Read the model definition and answer for the solid it produces. Units are mm, in the model's axes. Face numbers are marked on the shaded views. A direction names the side the tool comes from. Round coordinates to 2 decimals unless told otherwise and drop trailing zeros. Order: outer loops, then holes, each group sorted by start corner. A loop starts at its lowest first (then second) coordinate and runs counter-clockwise, first axis right, second up. Notation, with made-up numbers: (-23.5, -29.5) - (7.5, -29.5) arc R20 ccw to (7.5, -15.5) - close; hole circle Ø5 at (65, 89.25). An arc over 180 degrees is marked (long way). Answer as a JSON object with one key per item and string values. Group by question number.
Q1. The mould has two halves that part along Z. Classify the marked faces 1, 2 and 3: pulls with the +Z half, pulls with the -Z half, needs draft (parallel to the pull), parting line crosses it, or undercut.
Q2. A tool of negligible diameter and unlimited length cuts with its end or side. For the marked faces 4, 5, 6 and 7, from which of +Z, -Z, +X, -X, +Y, -Y can it reach the whole face along a straight path? Write none if from no direction.
Q3. Consider line 1 (Z direction, x = 53.9, y = 6.5); line 2 (Z direction, x = -8, y = 6); line 3 (X direction, y = 26, z = 4.5). Determine where each line is inside the solid, lowest interval first.
Q4. Given pin 1 Ø5 at (x, z) = (54, -1) entering from +Y; pin 2 Ø1.5 at (y, z) = (30.5, 29) entering from +X; pin 3 Ø20.5 at (x, z) = (17.5, 18.5) entering from -Y, each flat-ended and moving along its own axis, determine where each tip first touches the part or whether it passes through.
Q5. A cutting plane is placed at D-D on z = 23.5. Determine the outline of the cut face in (x, y).
Q6. A cutting plane is placed at C-C on x = 53.9. Determine the outline of the cut face in (y, z).
Q7. A cutting plane is placed at B-B on z = 14. Determine the outline of the cut face in (x, y), and give its area (3 significant figures).
```python
from build123d import *
from OCP.BRepFilletAPI import BRepFilletAPI_MakeFillet

# Parameters (mm, degrees)
SKETCH_1_W           = 71.9
SKETCH_1_H           = 40.1
SKETCH_1_W_2         = 4
SKETCH_1_H_2         = 1.4
SKETCH_1_H_3         = 0.9
EXTRUDE_1_DEPTH      = 35
SKETCH_4_W           = 8.4
SKETCH_4_H           = 4.4
SKETCH_4_W_2         = 30
SKETCH_4_H_2         = 2
CUT_EXTRUDE_2_DEPTH  = 77.710233998
SKETCH_5_W           = 71.9
SKETCH_5_H           = 40.1
EXTRUDE_2_DEPTH      = 3
SKETCH_6_W           = 47
SKETCH_6_H           = 0.9
CUT_EXTRUDE_3_DEPTH  = 79.124643999
SKETCH_7_R           = 1.6
CUT_EXTRUDE_4_DEPTH  = 79.124643999
SKETCH_10_W          = 10
SKETCH_10_H          = 39.2
SKETCH_10_H_2        = 40.1
CUT_EXTRUDE_6_DEPTH  = 35
CHAMFER_1_SIZE       = 10
CHAMFER_1_SIZE_2     = 11.917535926
SKETCH_8_R           = 3
CUT_EXTRUDE_5_DEPTH  = 35
SKETCH_11_W          = 17
SKETCH_11_H          = 32
CUT_EXTRUDE_7_DEPTH  = 2
CUT_EXTRUDE_8_DEPTH  = 79.124643999
FILLET_2_R1          = 2
FILLET_2_R2          = 3
SKETCH_13_W          = 24.9
SKETCH_13_H          = 1
EXTRUDE_3_DEPTH      = 38
SKETCH_14_W          = 11.9
SKETCH_14_H          = 1
CUT_EXTRUDE_9_DEPTH  = 35
CUT_EXTRUDE_10_REACH = 80.571
SKETCH_15_W          = 10
SKETCH_15_H          = 1
FILLET_3_R           = 3
FILLET_4_R           = 3
SKETCH_16_W          = 14.9
SKETCH_16_H          = 5.6
CUT_EXTRUDE_11_DEPTH = 35
FILLET_5_R           = 3


# Some blends are built 0.0001 mm under size
with BuildPart() as part:
    # 草图1 → 凸台-拉伸1 (new body)
    # profile 1 of 3: a face of its own
    with BuildSketch(Plane(origin=(0, 0, 0), x_dir=(1, 0, 0), z_dir=(0, 1, 0))):
        with Locations((22.95, -14.45)):
            Rectangle(SKETCH_1_W, SKETCH_1_H)
        Polygon((45.9, -32.5), (0, -32.5), (0, 0), (26.7, 0), (26.7, 2.6), (41.1, 2.6), (41.1, 0), (45.9, 0), align=None, mode=Mode.SUBTRACT)
    # profile 2 of 3: a face of its own
    with BuildSketch(Plane(origin=(0, 0, 0), x_dir=(1, 0, 0), z_dir=(0, 1, 0))):
        with Locations((2, -0.7)):
            Rectangle(SKETCH_1_W_2, SKETCH_1_H_2)
    # profile 3 of 3: a face of its own
    with BuildSketch(Plane(origin=(0, 0, 0), x_dir=(1, 0, 0), z_dir=(0, 1, 0))):
        with Locations((2, -32.05)):
            Rectangle(SKETCH_1_W_2, SKETCH_1_H_3)
    extrude(amount=EXTRUDE_1_DEPTH)

    # 草图4 → 切除-拉伸2 (cut, through all)
    with BuildSketch(Plane(origin=(0, 35, 0), x_dir=(1, 0, 0), z_dir=(0, 1, 0))):
        with Locations((10.12, 0.8)):
            Rectangle(SKETCH_4_W, SKETCH_4_H)
        with Locations((19, -33.5)):
            Rectangle(SKETCH_4_W_2, SKETCH_4_H_2)
    extrude(amount=-CUT_EXTRUDE_2_DEPTH, mode=Mode.SUBTRACT)

    # 草图5 → 凸台-拉伸2 (add)
    with BuildSketch(Plane(origin=(0, 35, 0), x_dir=(1, 0, 0), z_dir=(0, 1, 0))):
        with Locations((22.95, -14.45)):
            Rectangle(SKETCH_5_W, SKETCH_5_H)
    extrude(amount=EXTRUDE_2_DEPTH)

    # 草图6 → 切除-拉伸3 (cut, through all)
    with BuildSketch(Plane.XZ):
        with Locations((10.5, 34.05)):
            Rectangle(SKETCH_6_W, SKETCH_6_H)
    extrude(amount=-CUT_EXTRUDE_3_DEPTH, mode=Mode.SUBTRACT)

    # 草图7 → 切除-拉伸4 (cut, through all)
    with BuildSketch(Plane.XZ):
        with Locations(Location((-8, 27.5, 0), (0, 0, 270))):
            Circle(SKETCH_7_R)
        with Locations(Location((53.9, 27.5, 0), (0, 0, 270))):
            Circle(SKETCH_7_R)
        with Locations(Location((-8, -0.6, 0), (0, 0, 270))):
            Circle(SKETCH_7_R)
        with Locations(Location((53.9, -0.6, 0), (0, 0, 270))):
            Circle(SKETCH_7_R)
    extrude(amount=-CUT_EXTRUDE_4_DEPTH, mode=Mode.SUBTRACT)

    # 草图10 → 切除-拉伸6 (cut)
    with BuildSketch(Plane(origin=(0, 38, 0), x_dir=(1, 0, 0), z_dir=(0, 1, 0))):
        with Locations((-8, -14)):
            Rectangle(SKETCH_10_W, SKETCH_10_H)
        with Locations((53.9, -14.45)):
            Rectangle(SKETCH_10_W, SKETCH_10_H_2)
    extrude(amount=-CUT_EXTRUDE_6_DEPTH, mode=Mode.SUBTRACT)

    # 倒角1
    # the kernel refuses this chamfer: 11.917535926, 10 mm, written as the material it adds along each edge
    with BuildSketch(Plane(origin=(48.9, 3, -5.6), x_dir=(0.9993728857116146, -0.03540953691366307, 0), z_dir=(0, 0, 1))) as chamfer_1_piece_1_section:
        Polygon((CHAMFER_1_SIZE * 0.999372885712, CHAMFER_1_SIZE * 0.0354095369137), (-CHAMFER_1_SIZE_2 * 0.0354095369135, CHAMFER_1_SIZE_2 * 0.999372885707), (0, 0), align=None)
    chamfer_1_piece_1 = extrude(amount=40.1, mode=Mode.PRIVATE)
    chamfer_1_piece_1 = split(chamfer_1_piece_1, bisect_by=Plane(origin=(58.9, 6.996958781, 14.489120948), z_dir=(-1, 0, 0)), keep=Keep.TOP, mode=Mode.PRIVATE)
    chamfer_1_piece_1 = chamfer_1_piece_1 - Plane(origin=(53.9, 6.996958781, 27.5), x_dir=(0, 0, -1), z_dir=(0, -1, 0)) * Cylinder(1.6, 128, mode=Mode.PRIVATE)
    chamfer_1_piece_1 = chamfer_1_piece_1 - Plane(origin=(53.9, 6.996958781, -0.6), x_dir=(0, 0, -1), z_dir=(0, -1, 0)) * Cylinder(1.6, 128, mode=Mode.PRIVATE)
    add(chamfer_1_piece_1)
    with BuildSketch(Plane(origin=(-3, 3, -5.6), x_dir=(-0.9993728857116146, -0.03540953691366305, 0), z_dir=(0, 0, 1))) as chamfer_1_piece_2_section:
        Polygon((CHAMFER_1_SIZE * 0.999372885712, -CHAMFER_1_SIZE * 0.0354095369137), (-CHAMFER_1_SIZE_2 * 0.0354095369135, -CHAMFER_1_SIZE_2 * 0.999372885707), (0, 0), align=None)
    chamfer_1_piece_2 = extrude(amount=39.2, mode=Mode.PRIVATE)
    chamfer_1_piece_2 = split(chamfer_1_piece_2, bisect_by=Plane(origin=(-13, 6.997914765, 14.022030522), z_dir=(1, 0, 0)), keep=Keep.TOP, mode=Mode.PRIVATE)
    chamfer_1_piece_2 = chamfer_1_piece_2 - Plane(origin=(-8, 6.997914765, 27.5), x_dir=(0, 0, -1), z_dir=(0, -1, 0)) * Cylinder(1.6, 127, mode=Mode.PRIVATE)
    chamfer_1_piece_2 = chamfer_1_piece_2 - Plane(origin=(-8, 6.997914765, -0.6), x_dir=(0, 0, -1), z_dir=(0, -1, 0)) * Cylinder(1.6, 127, mode=Mode.PRIVATE)
    add(chamfer_1_piece_2)

    # 草图8 → 切除-拉伸5 (cut)
    with BuildSketch(Plane(origin=(0, 38, 0), x_dir=(1, 0, 0), z_dir=(0, 1, 0))):
        with Locations(Location((-8, 0.6, 0), (0, 0, 270))):
            Circle(SKETCH_8_R)
        with Locations(Location((53.9, 0.6, 0), (0, 0, 270))):
            Circle(SKETCH_8_R)
        with Locations(Location((53.9, -27.5, 0), (0, 0, 270))):
            Circle(SKETCH_8_R)
        with Locations(Location((-8, -27.5, 0), (0, 0, 270))):
            Circle(SKETCH_8_R)
    extrude(amount=-CUT_EXTRUDE_5_DEPTH, mode=Mode.SUBTRACT)

    # 草图11 → 切除-拉伸7 (cut)
    with BuildSketch(Plane.XY.offset(33.6)):
        with Locations((-4.5, 16)):
            Rectangle(SKETCH_11_W, SKETCH_11_H)
    extrude(amount=-CUT_EXTRUDE_7_DEPTH, mode=Mode.SUBTRACT)

    # 草图12 → 切除-拉伸8 (cut, through all)
    with BuildSketch(Plane(origin=(0, 38, 0), x_dir=(1, 0, 0), z_dir=(0, 1, 0))):
        Polygon((3, -2.4), (3, -25.6), (32.9, -2.4), align=None)
        Polygon((42.9, -2.4), (13, -25.6), (42.9, -25.6), align=None)
    extrude(amount=-CUT_EXTRUDE_8_DEPTH, mode=Mode.SUBTRACT)

    # 圆角2: one fillet with a radius per group of edges: ONE call of the kernel's fillet builder (fillet() takes one radius for all edges)
    fillet_2_edges_1 = [part.edges().sort_by_distance(p)[0] for p in [
        (13, 36.5, 25.6),
        (32.9, 36.5, 2.4),
    ]]
    fillet_2_edges_2 = [part.edges().sort_by_distance(p)[0] for p in [
        (3, 36.5, 25.6),
        (42.9, 36.5, 25.6),
        (42.9, 36.5, 2.4),
        (3, 36.5, 2.4),
    ]]
    fillet_2 = BRepFilletAPI_MakeFillet(part.part.solid().wrapped)
    for e in fillet_2_edges_1:
        fillet_2.Add(FILLET_2_R1, e.wrapped)
    for e in fillet_2_edges_2:
        fillet_2.Add(FILLET_2_R2, e.wrapped)
    add(Compound.cast(fillet_2.Shape()), mode=Mode.REPLACE)

    # 草图13 → 凸台-拉伸3 (add)
    with BuildSketch(Plane.XZ):
        with Locations((46.45, 35)):
            Rectangle(SKETCH_13_W, SKETCH_13_H)
    extrude(amount=-EXTRUDE_3_DEPTH)

    # 草图14 → 切除-拉伸9 (cut)
    with BuildSketch(Plane.XZ):
        with Locations((39.95, 33)):
            Rectangle(SKETCH_14_W, SKETCH_14_H)
    extrude(amount=-CUT_EXTRUDE_9_DEPTH, mode=Mode.SUBTRACT)

    # 切除-拉伸10: up to this face of the body (flat: up to its plane)
    cut_extrude_10_end = Plane(part.part.faces().sort_by_distance((53.9, 8.958767963, 14.614170269))[0])
    # 草图15 → 切除-拉伸10 (cut, up to the picked face)
    with BuildSketch(Plane(origin=(0, 38, 0), x_dir=(1, 0, 0), z_dir=(0, 1, 0)), mode=Mode.PRIVATE) as cut_extrude_10_sk1:
        with Locations((53.9, -35)):
            Rectangle(SKETCH_15_W, SKETCH_15_H)
    cut_extrude_10_tool1 = split(extrude(cut_extrude_10_sk1.sketch, amount=-CUT_EXTRUDE_10_REACH, mode=Mode.PRIVATE), bisect_by=cut_extrude_10_end, keep=Keep.BOTH, mode=Mode.PRIVATE)
    add(cut_extrude_10_tool1.solids().sort_by(Axis((53.9, 38, 35), (0, -1, 0)))[0], mode=Mode.SUBTRACT)

    # 圆角3
    fillet_3_edges = [part.edges().sort_by_distance(p)[0] for p in [
        (-3, 26.458767963, -5.6),
        (48.9, 26.458767963, -5.6),
        (48.9, 26.458767963, 35.5),
        (-3, 23.458767963, 31.6),
    ]]
    fillet(fillet_3_edges, radius=FILLET_3_R - 0.0001)  # a hair under: the kernel refuses the full size

    # 圆角4
    # the kernel refuses this fillet: 3 mm, written as the material it adds along each edge
    with BuildSketch(Plane(origin=(34, 35, 33.6), x_dir=(0, 0, 1), z_dir=(0, 1, 0))) as fillet_4_piece_1:
        with BuildLine():
            CenterArc((3, -2.791057147), FILLET_4_R, 111.510188267, 68.489811733)
            Line((0, -2.791057147), (-0.06, -2.791057147))
            Line((-0.06, -2.791057147), (-0.06, 0))
            Line((-0.06, 0), (0, 0.06))
            ThreePointArc((0, 0.06), (0.95, 0.06), (1.878, 0.055821143))
            Line((1.878, 0.055821143), (1.9, 0))
        make_face()
    extrude(amount=3)

    # 草图16 → 切除-拉伸11 (cut)
    with BuildSketch(Plane.XZ):
        with Locations((24.45, -2.8)):
            Rectangle(SKETCH_16_W, SKETCH_16_H)
    extrude(amount=-CUT_EXTRUDE_11_DEPTH, mode=Mode.SUBTRACT)

    # 圆角5
    fillet_5_edges = [part.edges().sort_by_distance(p)[0] for p in [
        (31.9, 17.5, -5.6),
        (17, 17.5, -5.6),
    ]]
    fillet(fillet_5_edges, radius=FILLET_5_R - 0.0001)  # a hair under: the kernel refuses the full size


solid = part.part
```
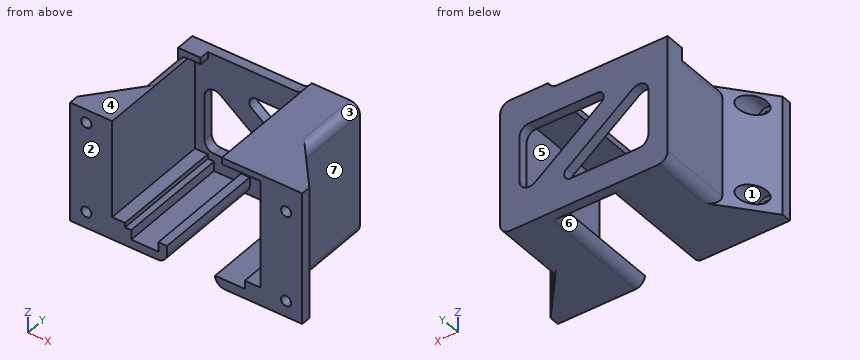
Result set:
{
 "1": {"face 1": "undercut", "face 2": "needs draft", "face 3": "pulls with the +Z half"},
 "2": {"face 4": "+Z, -X, -Y", "face 5": "-Y", "face 6": "-Z, -Y", "face 7": "+Z, -Z, +X, +Y"},
 "3": {"line 1": "z = -5.6 to -3.6, 2.4 to 24.5, 30.5 to 35.5", "line 2": "z = -5.6 to -3.6, 2.4 to 24.5, 30.5 to 31.6", "line 3": "x = -3 to 0, 45.9 to 48.9"},
 "4": {"pin 1": "stops at y = 3", "pin 2": "stops at x = 48.9", "pin 3": "stops at y = 35"},
 "5": {"outline": "(-13, 0) - (0, 0) - (0, 35) - (16.84, 35) - (16.84, 38) - (-3, 38) - (-3, 14.92) - (-13, 3) - close; (42.76, 35) - (45.9, 35) - (45.9, 0) - (58.9, 0) - (58.9, 3) - (48.9, 14.92) - (48.9, 38) - (42.76, 38) - close"},
 "6": {"outline": "(0, -5.6) - (8.96, -5.6) - (8.96, -3.6) - (3, -3.6) - (3, -2.2) - (0, -2.2) - close; (0, 1) - (3, 1) - (3, 2.4) - (8.96, 2.4) - (8.96, 24.5) - (3, 24.5) - (3, 25.9) - (0, 25.9) - close; (0, 29.1) - (3, 29.1) - (3, 30.5) - (8.96, 30.5) - (8.96, 35.5) - (0, 35.5) - close"},
 "7": {"outline": "(-13, 0) - (0, 0) - (0, 35) - (3, 35) - (3, 38) - (-3, 38) - (-3, 14.92) - (-13, 3) - close; (17.95, 35) - (27.95, 35) - (27.95, 38) - (17.95, 38) - close; (42.9, 35) - (45.9, 35) - (45.9, 0) - (58.9, 0) - (58.9, 3) - (48.9, 14.92) - (48.9, 38) - (42.9, 38) - close", "area": "455 mm²"}
}
